Check sheet for the modelled part. Datum: model origin and axes. Units: mm. Round coordinates to 2 decimals unless told otherwise and drop trailing zeros. Write each loop counter-clockwise with the first axis right and the second up, starting at its lowest first coordinate (ties: lowest second). Pieces come first, ordered by that corner, then holes. Notation, with made-up numbers: (74, 69) - (116, 69) arc R12 ccw to (116, 90) - close; hole circle Ø4 at (77, 27). An arc over 180 degrees is marked (long way). Use one line per item in the form item = value. Start each with the question number.
1) Section check A-A (z = 2.1). Record the boundary of the cut face in (x, y).
2) Scan lines: probe 1 along X at (y, z) = (58.5, 0.2); probe 2 along Y at (x, z) = (53, 0.6); probe 3 along Y at (x, z) = (51.5, 1.7). Record each from-to range of solid material in increasing order.
3) Gauge pin test, flat ends, axial feed: P1, Ø1.6, axis at x = 53.68, y = 87.04, coming from the +Z side; P2, Ø2.5, axis at x = 46.68, y = 80.04, coming from the -Z side; P3, Ø0.9, axis at y = -4, z = 1, coming from the +X side. Record the tip position at first contact, or that the pin passes through.
4) Section check C-C (x = -46.5). Record the boundary of the cut face in (y, z), then the cut area to 3 significant figures.
5) Section check B-B (y = 14). Record the boundary of the cut face in (x, z).
from build123d import *

# Parameters (mm, degrees)
EXTRUDE_1_DEPTH     = 3
SKETCH_2_R          = 1
CUT_EXTRUDE_1_DEPTH = 10
FILLET_1_R          = 4


with BuildPart() as part:
    # 草图1 → 凸台-拉伸1 (new body)
    with BuildSketch(Plane.XY):
        with BuildLine():
            Line((-60.568770688, -43.609385344), (-60.568770688, 100.290614656))
            Line((-60.568770688, 100.290614656), (33.431229312, 100.290614656))
            Line((33.431229312, 100.290614656), (46.681229312, 100.290614656))
            ThreePointArc((46.681229312, 100.290614656), (59.931229312, 87.040614656), (46.681229312, 73.790614656))
            Line((46.681229312, 73.790614656), (43.431229312, 73.790614656))
            ThreePointArc((43.431229312, 73.790614656), (36.3601615, 70.861682468), (33.431229312, 63.790614656))
            Line((33.431229312, 63.790614656), (33.431229312, -43.609385344))
            ThreePointArc((33.431229312, -43.609385344), (-13.568770688, -90.609385344), (-60.568770688, -43.609385344))
        make_face()
    extrude(amount=EXTRUDE_1_DEPTH)

    # 草图2 → 切除-拉伸1 (cut)
    with BuildSketch(Plane(origin=(0, 0, 0), x_dir=(-1, 0, 0), z_dir=(0, 0, -1))):
        with Locations((-46.681229312, 94.040614656)):
            Circle(SKETCH_2_R)
        with Locations((-39.681229312, 87.040614656)):
            Circle(SKETCH_2_R)
        with Locations((-46.681229312, 80.040614656)):
            Circle(SKETCH_2_R)
        with Locations((-53.681229312, 87.040614656)):
            Circle(SKETCH_2_R)
    extrude(amount=-CUT_EXTRUDE_1_DEPTH, mode=Mode.SUBTRACT)

    # 圆角1
    fillet_1_edges = [part.edges().sort_by_distance(p)[0] for p in [
        (-60.568770688, 100.290614656, 1.5),
    ]]
    fillet(fillet_1_edges, radius=FILLET_1_R)


solid = part.part
Results are:
q1.outline = (-60.57, -43.61) arc R47 ccw to (33.43, -43.61) - (33.43, 63.79) arc R10 cw to (43.43, 73.79) - (46.68, 73.79) arc R13.25 ccw to (46.68, 100.29) - (-56.57, 100.29) arc R4 ccw to (-60.57, 96.29) - close; hole circle Ø2 at (39.68, 87.04); hole circle Ø2 at (46.68, 80.04); hole circle Ø2 at (46.68, 94.04); hole circle Ø2 at (53.68, 87.04)
q2.probe_1 = -60.57 to 33.43
q2.probe_2 = 75.39 to 86.31, 87.77 to 98.69
q2.probe_3 = 74.7 to 99.38
q3.P1 = through
q3.P2 = 0
q3.P3 = 33.43
q4.outline = (-77.14, 0) - (100.29, 0) - (100.29, 3) - (-77.14, 3) - close
q4.area = 532 mm²
q5.outline = (-60.57, 0) - (33.43, 0) - (33.43, 3) - (-60.57, 3) - close
